from build123d import *

# Parameters (mm, degrees)
SKETCH1_R               = 13.5
BOSS_EXTRUDE1_DEPTH     = 3.5
CUT_EXTRUDE1_DEPTH      = 4.5
CUT_EXTRUDE1_DEPTH_BACK = 4.5
CHAMFER1_SIZE           = 1
M16_TAPPED_HOLE1_D      = 14
M16_TAPPED_HOLE1_DEPTH  = 7


with BuildPart() as part:
    # Sketch1 → Boss-Extrude1 (new body, symmetric)
    with BuildSketch(Plane(origin=(0, 0, 0), x_dir=(1, 0, 0), z_dir=(0, 1, 0))):
        Circle(SKETCH1_R)
    extrude(amount=BOSS_EXTRUDE1_DEPTH, both=True)

    # Sketch2 → Cut-Extrude1 (cut, two sides)
    with BuildSketch(Plane(origin=(0, 0, 0), x_dir=(1, 0, 0), z_dir=(0, 1, 0))) as cut_extrude1_sk:
        with BuildLine():
            Line((-2, 13.351029923), (-2, 11.351029923))
            Line((-2, 11.351029923), (2, 11.351029923))
            Line((2, 11.351029923), (2, 13.351029923))
            ThreePointArc((2, 13.351029923), (0, 13.5), (-2, 13.351029923))
        make_face()
        with BuildLine():
            Line((13.351029923, 2), (11.351029923, 2))
            Line((11.351029923, 2), (11.351029923, -2))
            Line((11.351029923, -2), (13.351029923, -2))
            ThreePointArc((13.351029923, -2), (13.5, 0), (13.351029923, 2))
        make_face()
        with BuildLine():
            Line((2, -13.351029923), (2, -11.351029923))
            Line((2, -11.351029923), (-2, -11.351029923))
            Line((-2, -11.351029923), (-2, -13.351029923))
            ThreePointArc((-2, -13.351029923), (0, -13.5), (2, -13.351029923))
        make_face()
        with BuildLine():
            Line((-13.351029923, -2), (-11.351029923, -2))
            Line((-11.351029923, -2), (-11.351029923, 2))
            Line((-11.351029923, 2), (-13.351029923, 2))
            ThreePointArc((-13.351029923, 2), (-13.5, 0), (-13.351029923, -2))
        make_face()
    extrude(amount=CUT_EXTRUDE1_DEPTH, mode=Mode.SUBTRACT)
    extrude(cut_extrude1_sk.sketch, amount=-CUT_EXTRUDE1_DEPTH_BACK, mode=Mode.SUBTRACT)

    # Chamfer1
    chamfer1_edges = [part.edges().sort_by_distance(p)[0] for p in [
        (9.545941546, 3.5, -9.545941546),
        (-9.545941546, 3.5, -9.545941546),
        (-9.545941546, 3.5, 9.545941546),
        (9.545941546, 3.5, 9.545941546),
    ]]
    chamfer(chamfer1_edges, length=CHAMFER1_SIZE)

    # M16 Tapped Hole1
    with Locations(Plane(origin=(0, 3.5, 0), x_dir=(1, 0, 0), z_dir=(0, 1, 0))):
        with Locations((0, 0)):
            Hole(M16_TAPPED_HOLE1_D / 2, depth=M16_TAPPED_HOLE1_DEPTH)


solid = part.part
Build history of the part. All positions in model axes, mm. A direction names the side the tool comes from. Coordinates: 2 decimals unless noted, no trailing zeros. Write each loop counter-clockwise with the first axis right and the second up, starting at its lowest first coordinate (ties: lowest second). Pieces come first, ordered by that corner, then holes. Notation, with made-up numbers: (-7, 13) -> (47, 13) arc R10 ccw to (47, 28) -> close; hole circle Ø8 at (42, 20.25). An arc over 180 degrees is marked (long way). Use CSV: the item, a comma, the result in double quotes. Start each with the question number.
Q1. Drill centre lines: probe 1 along Z at (x, y) = (0, 1.5); probe 2 along Z at (x, y) = (-5.75, 3); probe 3 along X at (y, z) = (2.25, 3.75). Where is each one in solid material? Low to high.
Q2. Cut at B-B, the plane y = -2.75. List the corners of the cut face in (x, z), then the cut area to 3 significant figures.
Q3. 3-axis set-ups, long thin cutter, end or side, ignore diameter. For faces 5 (the flat face through (-12, 0, -2)), 6 (the flat face through (2, 0, 12)), 7 (the flat face through (11.351, 0, 0)), 8 (the flat face through (0, 0, -11.351)): which of +Z, -Z, +X, -X, +Y, -Y reach the whole face in a straight line?
Q4. Cut at C-C, the plane x = 0. List the corners of the cut face in (y, z).
Q5. Flat gauge pins, fed straight in: pin 1 Ø1 at (y, z) = (-1.5, 13) entering from -X; pin 2 Ø2 at (x, y) = (12.5, -0.5) entering from -Z; pin 3 Ø0.6 at (y, z) = (0.5, -12) entering from +X (3 decimals). Where does each tip first touch, or does it go through?
Q6. Cut at A-A, the plane z = 0. List the corners of the cut face in (x, y), then the cut area to 3 significant figures.
Q7. Pull direction Z, two halves, no side cores. Call faces 1 (the flat face through (12, 0, -2)), 2 (the flat face through (-2, 0, -12)), 3 (the conical face through (-8.87, 3.34, -9.03)), 4 (the conical face through (8.87, 3.34, 9.03)): released by +Z, released by -Z, zero draft, split by the parting line, or undercut.
Checked values:
1,probe 1,"z = -11.35 to -7, 7 to 11.35"
1,probe 2,"z = -11.66 to -3.99, 3.99 to 11.66"
1,probe 3,"x = -12.97 to -5.91, 5.91 to 12.97"
2,outline,"(-13.35, -2) arc R13.5 ccw to (-2, -13.35) -> (-2, -11.35) -> (2, -11.35) -> (2, -13.35) arc R13.5 ccw to (13.35, -2) -> (11.35, -2) -> (11.35, 2) -> (13.35, 2) arc R13.5 ccw to (2, 13.35) -> (2, 11.35) -> (-2, 11.35) -> (-2, 13.35) arc R13.5 ccw to (-13.35, 2) -> (-11.35, 2) -> (-11.35, -2) -> close; hole circle Ø14 at (0, 0)"
2,area,"385 mm²"
3,face 5,"-X, +Y, -Y"
3,face 6,"+Z, +Y, -Y"
3,face 7,"+X, +Y, -Y"
3,face 8,"-Z, +Y, -Y"
4,outline,"(-3.5, -11.35) -> (3.5, -11.35) -> (3.5, -7) -> (-3.5, -7) -> close; (-3.5, 7) -> (3.5, 7) -> (3.5, 11.35) -> (-3.5, 11.35) -> close"
5,pin 1,"stops at x = -5.1"
5,pin 2,"stops at z = -7.07"
5,pin 3,"stops at x = 6.735"
6,outline,"(-11.35, -3.5) -> (-7, -3.5) -> (-7, 3.5) -> (-11.35, 3.5) -> close; (7, -3.5) -> (11.35, -3.5) -> (11.35, 3.5) -> (7, 3.5) -> close"
6,area,"60.9 mm²"
7,face 1,"undercut"
7,face 2,"zero draft"
7,face 3,"released by -Z"
7,face 4,"released by +Z"
